Work out the finished part from the listing and answer in its coordinate system (mm). A direction names the side the tool comes from. Round coordinates to 2 decimals unless told otherwise and drop trailing zeros. Order: outer loops, then holes, each group sorted by start corner. A loop starts at its lowest first (then second) coordinate and runs counter-clockwise, first axis right, second up. Notation, with made-up numbers: (11, -39) - (26, -39) arc R22 cw to (26, -17) - close; hole circle Ø3 at (32.5, -25.75). An arc over 180 degrees is marked (long way). Use one line per item in the form item = value. Start each with the question number.
Q1. The part is cut by section B-B on z = 6. Determine the outline of the cut face in (x, y), plus the area to 3 significant figures.
Q2. Given P1, Ø1.5, axis at y = 3.5, z = 19.5, coming from the -X side; P2, Ø3, axis at y = 7.5, z = 11.5, coming from the -X side, each flat-ended and moving along its own axis, determine where each tip first touches the part or whether it passes through.
Q3. The part is cut by section A-A on y = 0. Determine the outline of the cut face in (x, z).
Q4. The part is cut by section D-D on z = -11.5. Determine the outline of the cut face in (x, y).
Q5. Which of the six approach directions +Z, -Z, +X, -X, +Y, -Y give full straight-line access (tool end or side, diameter ignored) to faces 1 (the flat face through (-5, 5, 46.99)), 2 (the cylindrical face through (-4.21, -18.97, 23.17))?
Q6. For a pull along X with two mould halves and no side action, classify faces 3 (the cylindrical face through (-22.071, -16.924, 6.026)), 4 (the flat face through (0, 7, -16.51)), 5 (the cylindrical face through (-1.404, -6.323, 14.796)) as +X half, -X half, draft (parallel to the pull), parting line (faces both ways), or undercut.
Q7. Find the intervals of material crossed by line 1 (Y direction, x = 0, z = 15); line 2 (Y direction, x = 3.5, z = 1); line 3 (X direction, y = -14.5, z = 17.5), in increasing order. Write a range as [from, to].
from build123d import *

# Parameters (mm, degrees)
F0_R     = 27.813
F0_R_2   = 24.6126
F1_DEPTH = 27.94
F0_R_3   = 19.431
F0_R_4   = 6.477
F2_DEPTH = 16.51
F3_DEPTH = 19.05


with BuildPart() as f1:
    # F0 (on Top) → F1 (new body)
    with BuildSketch(Plane.XY):
        Circle(F0_R)
        Circle(F0_R_2, mode=Mode.SUBTRACT)
    extrude(amount=F1_DEPTH)



with BuildPart() as f1b:
    # F0 (on Top) → F1, piece 2 (new body)
    with BuildSketch(Plane.XY):
        Circle(F0_R_3)
        Circle(F0_R_4, mode=Mode.SUBTRACT)
    extrude(amount=F1_DEPTH)


with BuildPart() as f1_1:
    add(f1.part)

    add(f1b.part)  # F2 merges F1b
    # F0 (on Top) → F2 (join)
    with BuildSketch(Plane.XY):
        Circle(F0_R)
        Circle(F0_R_2, mode=Mode.SUBTRACT)
        Circle(F0_R_2)
        Circle(F0_R_3, mode=Mode.SUBTRACT)
        Circle(F0_R_3)
        Circle(F0_R_4, mode=Mode.SUBTRACT)
    extrude(amount=-F2_DEPTH)

    # F3 (add): a face of the model
    f3_faces = [f1_1.faces().sort_by_distance(p)[0] for p in [
        (-18.8814083254, 0, 27.94),
    ]]
    extrude(f3_faces, amount=F3_DEPTH)


solid = f1_1.part
Found:
q1.outline = circle Ø55.63 at (0, 0); circle Ø38.86 at (0, 0); hole circle Ø49.23 at (0, 0); hole circle Ø12.95 at (0, 0)
q1.area = 1,580 mm²
q2.P1 = -27.68
q2.P2 = -27.16
q3.outline = (-27.81, -16.51) - (-6.48, -16.51) - (-6.48, 46.99) - (-19.43, 46.99) - (-19.43, 0) - (-24.61, 0) - (-24.61, 27.94) - (-27.81, 27.94) - close; (6.48, -16.51) - (27.81, -16.51) - (27.81, 27.94) - (24.61, 27.94) - (24.61, 0) - (19.43, 0) - (19.43, 46.99) - (6.48, 46.99) - close
q4.outline = circle Ø55.63 at (0, 0); hole circle Ø12.95 at (0, 0)
q5.face_1 = +Z, +X, -X, +Y, -Y
q5.face_2 = +Z
q6.face_3 = parting line
q6.face_4 = draft
q6.face_5 = undercut
q7.line_1 = [-27.81, -24.61], [-19.43, -6.48], [6.48, 19.43], [24.61, 27.81]
q7.line_2 = [-27.59, -24.36], [-19.11, -5.45], [5.45, 19.11], [24.36, 27.59]
q7.line_3 = [-23.73, -19.89], [-12.93, 12.93], [19.89, 23.73]
